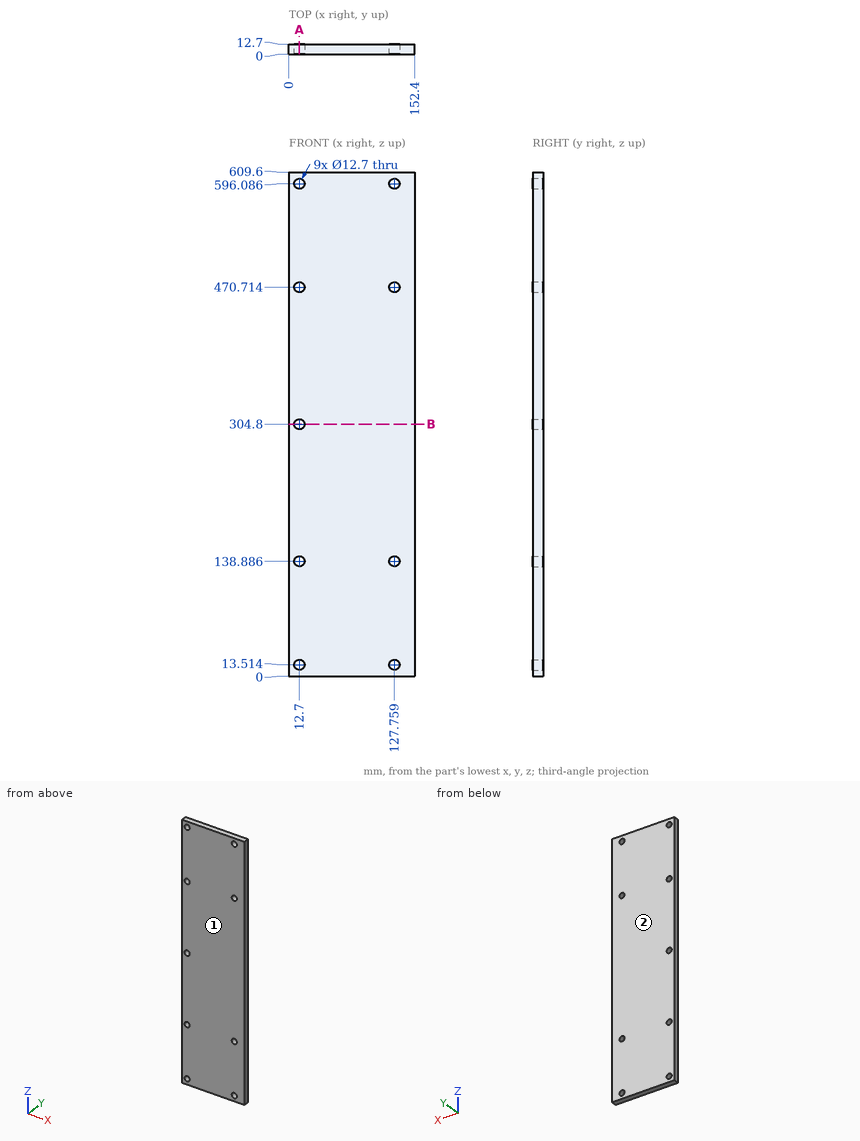
Geometry check sheet. Reference: drawing and pictorial views, mm from the part's lowest x, y, z. Coordinates: 2 decimals unless noted, no trailing zeros. Loops run counter-clockwise (first coordinate to the right, second up) from the corner with the lowest first, then second, coordinate; pieces in that order, holes last. Notation, with made-up numbers: (85, 18) -> (113, 18) arc R24 cw to (113, 48) -> close; hole circle Ø9 at (-13.75, -15). An arc over 180 degrees is marked (long way). Write item = value, one per line. Start each with the question number.
1. Draft check along Y on the marked faces 1 and 2. Enter one of: released by +Y, released by -Y, zero draft, split by the parting line, or undercut.
2. Section check A-A on x = 12.7. Record the cut outline in (y, z).
3. Material ranges on line 1 (Z direction, x = 12.7, y = 5); line 2 (Z direction, x = 124, y = 5.5) (1 decimal); line 3 (X direction, y = 7.75, z = 141), recorded low to high.
4. Depth check by flat-ended pin: P1, Ø11.5, axis at x = 12.7, z = 13.51, coming from the +Y side; P2, Ø2, axis at x = 91, y = 8, coming from the -Z side. Enter the tip coordinate at first touch or a pass-through.
5. Section check B-B on z = 304.8. Record the cut outline in (x, y), then the cut area to 3 significant figures.
Responses:
q1.face_1 = released by -Y
q1.face_2 = released by +Y
q2.outline = (0, 0) -> (12.7, 0) -> (12.7, 7.16) -> (0, 7.16) -> close; (0, 19.86) -> (12.7, 19.86) -> (12.7, 132.54) -> (0, 132.54) -> close; (0, 145.24) -> (12.7, 145.24) -> (12.7, 298.45) -> (0, 298.45) -> close; (0, 311.15) -> (12.7, 311.15) -> (12.7, 464.36) -> (0, 464.36) -> close; (0, 477.06) -> (12.7, 477.06) -> (12.7, 589.74) -> (0, 589.74) -> close; (0, 602.44) -> (12.7, 602.44) -> (12.7, 609.6) -> (0, 609.6) -> close
q3.line_1 = 0 to 7.16, 19.86 to 132.54, 145.24 to 298.45, 311.15 to 464.36, 477.06 to 589.74, 602.44 to 609.6
q3.line_2 = 0 to 8.4, 18.6 to 133.8, 144 to 465.6, 475.8 to 591, 601.2 to 609.6
q3.line_3 = 0 to 6.71, 18.69 to 121.77, 133.75 to 152.4
q4.P1 = through
q4.P2 = 0
q5.outline = (0, 0) -> (6.35, 0) -> (6.35, 12.7) -> (0, 12.7) -> close; (19.05, 0) -> (152.4, 0) -> (152.4, 12.7) -> (19.05, 12.7) -> close
q5.area = 1,770 mm2
